```python
from build123d import *

# Parameters (mm, degrees)
SKETCH2_R          = 1.75
CUT_EXTRUDE1_DEPTH = 17
CIRPATTERN1_COUNT  = 2
CIRPATTERN1_ANGLE  = 90
CHAMFER1_SIZE      = 0.6


with BuildPart() as part:
    # Sketch1 → Revolve1 (revolve)
    with BuildSketch(Plane.XY):
        Polygon((-10.58638484, 3.995), (-7.464927114, 3.995), (-1.431661808, 3.995), (15.33361516, 3.995), (15.33361516, 11.005), (13.83361516, 11.005), (13.83361516, 9.11), (-2.16638484, 9.11), (-2.16638484, 11.005), (-10.58638484, 11.005), align=None)
    revolve(axis=Axis((0, 0, 0), (1, 0, 0)))

    # Sketch2 → Cut-Extrude1 (cut)
    with BuildSketch(Plane.XY):
        with Locations((-6.37638484, 0)):
            Circle(SKETCH2_R)
    cut_extrude1 = extrude(amount=-CUT_EXTRUDE1_DEPTH, mode=Mode.SUBTRACT)

    # CirPattern1: Cut-Extrude1 ×2 about axis
    cirpattern1_axis = Axis((-10.58638484, 0, 0), (-1, 0, 0))
    for i in range(1, CIRPATTERN1_COUNT):
        add(cut_extrude1.rotate(cirpattern1_axis, i * CIRPATTERN1_ANGLE / (CIRPATTERN1_COUNT - 1)), mode=Mode.SUBTRACT)

    # Chamfer1
    chamfer1_edges = [part.edges().sort_by_distance(p)[0] for p in [
        (-2.16638484, -11.005, 0),
        (13.83361516, -11.005, 0),
    ]]
    chamfer(chamfer1_edges, length=CHAMFER1_SIZE)


solid = part.part
```
The listing builds one solid part. Answer for the finished solid, in the listing's coordinates (mm). A direction names the side the tool comes from. Coordinates: 2 decimals unless noted, no trailing zeros. Write each loop counter-clockwise with the first axis right and the second up, starting at its lowest first coordinate (ties: lowest second). Pieces come first, ordered by that corner, then holes. Notation, with made-up numbers: (-2.5, -20) - (19.5, -20) arc R20 ccw to (19.5, -12) - close; hole circle Ø1 at (-28, 56). An arc over 180 degrees is marked (long way). Return JSON: item names as keys, results as strings. Group by question number.
1. Given pin 1 (10.5 mm diameter, centred on y = -2.5, z = -1.5, fed in from +X); pin 2 (10 mm diameter, centred on x = 9, z = 2.5, fed in from +Y); pin 3 (1 mm diameter, centred on x = -3.5, y = 2, fed in from -Z); pin 4 (8 mm diameter, centred on x = 7, y = 7.5, fed in from -Z), each flat-ended and moving along its own axis, determine where each tip first touches the part or whether it passes through.
2. Determine the mould class of faces 4 (the cylindrical face through (14.9, 10.5, 3.3)), 5 (the flat face through (-10.586, 5, 0)), 6 (the cylindrical face through (5.722, 4.204, -8.082)) for opening direction X: released by +X, released by -X, zero draft, split by the parting line, or undercut.
3. Straight lines are drawn through the part: L1, parallel to Z at x = -4, y = 0 (3 decimals); L2, parallel to Z at x = 0, y = 0 (3 decimals); L3, parallel to X at y = 0, z = -6.5. For each, find the intervals that lie inside material, in ascending order.
4. A cutting plane is placed at C-C, the plane x = -4. Determine the outline of the cut face in (y, z) (3 decimals), plus the area to 3 significant figures.
5. Which of the six approach directions +Z, -Z, +X, -X, +Y, -Y give full straight-line access (tool end or side, diameter ignored) to faces 1 (the cylindrical face through (-5.569, -1.553, -7.248)), 2 (the cylindrical face through (-5.569, -7.246, 1.553)), 3 (the flat face through (13.834, 5, -8))?
6. A cutting plane is placed at A-A, the plane y = 0. Determine the outline of the cut face in (x, z) (3 decimals).
7. A cutting plane is placed at D-D, the plane x = 9.75. Determine the outline of the cut face in (y, z) (3 decimals), plus the area to 3 significant figures.
Ans:
{
 "1": {"pin 1": "x = 15.33", "pin 2": "y = 10.37", "pin 3": "z = -10.9", "pin 4": "z = -8.41"},
 "2": {"face 4": "zero draft", "face 5": "released by -X", "face 6": "undercut"},
 "3": {"L1": "-11.005 to -3.995, 3.995 to 11.005", "L2": "-9.11 to -3.995, 3.995 to 9.11", "L3": "-10.59 to -8.13, -4.63 to 15.33"},
 "4": {"outline": "circle Ø22.01 at (0, 0); hole circle Ø7.99 at (0, 0)", "area": "330 mm²"},
 "5": {"face 1": "-Z", "face 2": "-Y", "face 3": "none"},
 "6": {"outline": "(-10.586, -11.005) - (-8.126, -11.005) - (-8.126, -3.995) - (-10.586, -3.995) - close; (-10.586, 3.995) - (15.334, 3.995) - (15.334, 11.005) - (14.434, 11.005) - (13.834, 10.405) - (13.834, 9.11) - (-2.166, 9.11) - (-2.166, 10.405) - (-2.766, 11.005) - (-10.586, 11.005) - close; (-4.626, -11.005) - (-2.766, -11.005) - (-2.166, -10.405) - (-2.166, -9.11) - (13.834, -9.11) - (13.834, -10.405) - (14.434, -11.005) - (15.334, -11.005) - (15.334, -3.995) - (-4.626, -3.995) - close"},
 "7": {"outline": "circle Ø18.22 at (0, 0); hole circle Ø7.99 at (0, 0)", "area": "211 mm²"}
}
